```python
from build123d import *

# Parameters (mm, degrees)
SKETCH1_W           = 85
SKETCH1_H           = 10
SKETCH1_R           = 2
BOSS_EXTRUDE1_DEPTH = 2
CUT_EXTRUDE1_DEPTH  = 10
SKETCH3_W           = 15
SKETCH3_H           = 10
BOSS_EXTRUDE2_DEPTH = 13
BOSS_EXTRUDE3_DEPTH = 10
BOSS_EXTRUDE4_DEPTH = 10


with BuildPart() as part:
    # Sketch1 → Boss-Extrude1 (new body)
    with BuildSketch(Plane(origin=(0, 0, 0), x_dir=(1, 0, 0), z_dir=(0, 1, 0))):
        with Locations((18.270818553, 2.053936679)):
            Rectangle(SKETCH1_W, SKETCH1_H)
        with Locations(Location((-19.229181447, 2.053936679, 0), (0, 0, 270))):
            Circle(SKETCH1_R, mode=Mode.SUBTRACT)
        with Locations(Location((5.770818553, 2.053936679, 0), (0, 0, 270))):
            Circle(SKETCH1_R, mode=Mode.SUBTRACT)
    extrude(amount=BOSS_EXTRUDE1_DEPTH)

    # Sketch2 → Cut-Extrude1 (cut)
    with BuildSketch(Plane(origin=(0, 2, 0), x_dir=(1, 0, 0), z_dir=(0, 1, 0))):
        Polygon((60.770818553, 2.053936679), (55.770818553, -2.946063321), (60.770818553, -2.946063321), align=None)
    extrude(amount=-CUT_EXTRUDE1_DEPTH, mode=Mode.SUBTRACT)

    # Sketch3 → Boss-Extrude2 (add)
    with BuildSketch(Plane(origin=(29.358440937, 0, 29.358440937), x_dir=(0.7071067811865439, 0, -0.7071067811865511), z_dir=(0.7071067811865511, 0, 0.7071067811865439))):
        with Locations((38.590339713, 0.888307249)):
            Rectangle(SKETCH3_W, SKETCH3_H)
    extrude(amount=BOSS_EXTRUDE2_DEPTH)

    # Sketch4 → Boss-Extrude3 (add)
    with BuildSketch(Plane(origin=(0, 5.888307249, 0), x_dir=(1, 0, 0), z_dir=(0, 1, 0))):
        Polygon((51.342630977, -7.374250897), (49.762527896, -2.752596668), (55.964285206, -2.752596668), align=None)
    extrude(amount=-BOSS_EXTRUDE3_DEPTH)

    # Sketch5 → Boss-Extrude4 (add)
    with BuildSketch(Plane(origin=(0, 5.888307249, 0), x_dir=(1, 0, 0), z_dir=(0, 1, 0))):
        Polygon((71.141620851, -5.960037335), (71.141620851, -6.460037335), (70.641620851, -6.460037335), align=None)
        Polygon((70.434514069, -6.667144116), (70.434514069, -7.167144116), (69.934514069, -7.167144116), align=None)
        Polygon((69.727407288, -7.374250897), (69.727407288, -7.874250897), (69.227407288, -7.874250897), align=None)
        Polygon((69.020300507, -8.081357678), (69.020300507, -8.581357678), (68.520300507, -8.581357678), align=None)
        Polygon((68.313193726, -8.788464459), (68.313193726, -9.288464459), (67.813193726, -9.288464459), align=None)
        Polygon((67.606086945, -9.495571241), (67.606086945, -9.995571241), (67.106086945, -9.995571241), align=None)
        Polygon((66.898980164, -10.202678022), (66.898980164, -10.702678022), (66.398980164, -10.702678022), align=None)
        Polygon((66.191873382, -10.909784803), (66.191873382, -11.409784803), (65.691873382, -11.409784803), align=None)
        Polygon((65.484766601, -11.616891584), (65.484766601, -12.116891584), (64.984766601, -12.116891584), align=None)
        Polygon((64.77765982, -12.323998365), (64.77765982, -12.823998365), (64.27765982, -12.823998365), align=None)
        Polygon((64.070553039, -13.031105147), (64.070553039, -13.531105147), (63.570553039, -13.531105147), align=None)
        Polygon((63.363446258, -13.738211928), (63.363446258, -14.238211928), (62.863446258, -14.238211928), align=None)
        Polygon((62.656339476, -14.445318709), (62.656339476, -14.945318709), (62.156339476, -14.945318709), align=None)
        Polygon((61.949232695, -15.15242549), (61.949232695, -15.65242549), (61.449232695, -15.65242549), align=None)
        Polygon((61.242125914, -15.859532271), (61.242125914, -16.359532271), (60.742125914, -16.359532271), align=None)
    extrude(amount=-BOSS_EXTRUDE4_DEPTH)


solid = part.part
```
Geometry: final body of the model. Coordinates: model frame, mm. A direction names the side the tool comes from. Coordinates: 2 decimals unless noted, no trailing zeros. Loops run counter-clockwise (first coordinate to the right, second up) from the corner with the lowest first, then second, coordinate; pieces in that order, holes last. Notation, with made-up numbers: (-29, -15.5) -> (-8, -15.5) arc R19 cw to (-8, 7.5) -> close; hole circle Ø9 at (-13, -21). An arc over 180 degrees is marked (long way). Use a Markdown table: item, result. Add a question column.
(1) Section query B-B, the plane z = -5. Return loops of the section in (x, y), plus the area to 3 significant figures.
(2) Pin query (flat end, axial travel): pin 1 Ø2 at (x, y) = (52.5, -1.5) entering from -Z; pin 2 Ø5 at (y, z) = (-0.5, 14) entering from -X; pin 3 Ø0.6 at (y, z) = (1, 13) entering from +X. Return the tip coordinate at first contact, or that it passes through.
(3) Section query D-D, the plane z = 1.5. Return loops of the section in (x, y), plus the area to 3 significant figures.
(4) Section query A-A, the plane x = 55. Return loops of the section in (y, z).
(5) Access query for faces 1 (the flat face through (66.48, 0.82, 1.3)), 2 (the flat face through (12, 1, 2.946)), 3 (the flat face through (53, -2, 2.753)). Directions: +Z, -Z, +X, -X, +Y, -Y. A direction counts if a zero-diameter tool reaches every point of the face in a straight line with its end or side. Return the directions, or none.
(6) Section query C-C, the plane x = -7. Return loops of the section in (y, z), plus the area to 3 significant figures.
(7) Mould query, pull axis X, two halves, no side actions, for faces 4 (the flat face through (53, 4, 2.753)), 5 (the cylindrical face through (-17.54, 0.99, -0.98)), 6 (the flat face through (55.874, 0.818, 11.906)). Classes: pulls with the +X half, pulls with the -X half, needs draft (parallel to the pull), parting line crosses it, or undercut.
(8) Line query: line 1 along Z through (x, y) = (40, 1.5); line 2 along X through (y, z) = (0.5, -0.5); line 3 along Y through (x, z) = (53.5, -5.25). Output: solid intervals per line, ascending.
Answer:
| question | item | result |
|---|---|---|
| 1 | outline | (-24.23, 0) -> (60.77, 0) -> (60.77, 2) -> (-24.23, 2) -> close |
| 1 | area | 170 mm^2 |
| 2 | pin 1 | stops at z = 2.75 |
| 2 | pin 2 | stops at x = 55.47 |
| 2 | pin 3 | stops at x = 64.78 |
| 3 | outline | (-24.23, 0) -> (57.22, 0) -> (57.22, -4.11) -> (66.68, -4.11) -> (66.68, 5.89) -> (57.22, 5.89) -> (57.22, 2) -> (-24.23, 2) -> close |
| 3 | area | 258 mm^2 |
| 4 | outline | (-4.11, 2.75) -> (0, 2.75) -> (0, -7.05) -> (2, -7.05) -> (2, 2.75) -> (5.89, 2.75) -> (5.89, 11.03) -> (-4.11, 11.03) -> close |
| 5 | face 1 | -Z, +X, +Y, -Y |
| 5 | face 2 | +Z, -X, +Y, -Y |
| 5 | face 3 | -Z, -X, -Y |
| 6 | outline | (0, -7.05) -> (2, -7.05) -> (2, 2.95) -> (0, 2.95) -> close |
| 6 | area | 20.0 mm^2 |
| 7 | face 4 | needs draft |
| 7 | face 5 | undercut |
| 7 | face 6 | pulls with the -X half |
| 8 | line 1 | z = -7.05 to 2.95 |
| 8 | line 2 | x = -24.23 to -20.49, -17.97 to 4.51, 7.03 to 64.68 |
| 8 | line 3 | y = 0 to 2 |
